Autodesk Inventor part; units mm, degrees
ref_plane "Startebene" through (0, 0, 0) normal (0, 0, 1) x (1, 0, 0)
ref_plane "Endebene" through (0, 0, 100) normal (0, 0, 1) x (1, 0, 0)
ref_plane "YZ Plane" through (0, 0, 0) normal (1, 0, 0) x (0, 1, 0)
ref_plane "Startebene" through (0, 0, 0) normal (0, 0, 1) x (1, 0, 0)
ref_plane "Endebene" through (0, 0, 100) normal (0, 0, 1) x (1, 0, 0)
sketch "Skizze" plane through (0, 0, 0) normal (0, 0, 1) x (1, 0, 0)
  arc A0 (-4.5287, -3.2559) -> (-3.65, -1.1346) centre (-6.65, -1.1346) ccw
  line L0 (-3.65, -1.1346) -> (-3.65, 1.1346)
  circle A1 centre (0, 0) radius 2.15
  line L1 (1.1346, -3.65) -> (-1.1346, -3.65)
  arc A2 (-1.1346, -3.65) -> (-3.2559, -4.5287) centre (-1.1346, -6.65) ccw
  line L2 (-6.779, -5.5062) -> (-4.5287, -3.2559)
  line L3 (-3.2559, -4.5287) -> (-5.5062, -6.779)
  arc A3 (-2.5, -8.5) -> (-2.8, -8.2) centre (-2.8, -8.5) ccw
  line L4 (-2.5, -8.5) -> (-2.5, -9.2)
  line L5 (-4.9176, -8.2) -> (-2.8, -8.2)
  arc A4 (-5.5062, -6.779) -> (-4.9176, -8.2) centre (-4.9176, -7.3676) ccw
  arc A5 (-3.3, -10) -> (-2.5, -9.2) centre (-3.3, -9.2) ccw
  line L6 (-3.3, -10) -> (-8, -10)
  line L7 (10, -3.3) -> (10, -8)
  line L8 (5.5062, -6.779) -> (3.2559, -4.5287)
  arc A6 (6.779, -5.5062) -> (8.2, -4.9176) centre (7.3676, -4.9176) ccw
  arc A7 (3.2559, -4.5287) -> (1.1346, -3.65) centre (1.1346, -6.65) ccw
  line L9 (4.5287, -3.2559) -> (6.779, -5.5062)
  arc A8 (3.65, -1.1346) -> (4.5287, -3.2559) centre (6.65, -1.1346) ccw
  arc A9 (8.5, -2.5) -> (8.2, -2.8) centre (8.5, -2.8) ccw
  line L10 (3.65, 1.1346) -> (3.65, -1.1346)
  line L11 (8.5, -2.5) -> (9.2, -2.5)
  arc A10 (10, -3.3) -> (9.2, -2.5) centre (9.2, -3.3) ccw
  line L12 (8.2, -4.9176) -> (8.2, -2.8)
  line L13 (2.5, 8.5) -> (2.5, 9.2)
  arc A11 (2.5, 8.5) -> (2.8, 8.2) centre (2.8, 8.5) ccw
  arc A12 (1.1346, 3.65) -> (3.2559, 4.5287) centre (1.1346, 6.65) ccw
  line L14 (-1.1346, 3.65) -> (1.1346, 3.65)
  arc A13 (3.3, 10) -> (2.5, 9.2) centre (3.3, 9.2) ccw
  line L15 (4.9176, 8.2) -> (2.8, 8.2)
  arc A14 (4.5287, 3.2559) -> (3.65, 1.1346) centre (6.65, 1.1346) ccw
  line L16 (3.2559, 4.5287) -> (5.5062, 6.779)
  arc A15 (5.5062, 6.779) -> (4.9176, 8.2) centre (4.9176, 7.3676) ccw
  line L17 (6.779, 5.5062) -> (4.5287, 3.2559)
  line L18 (3.3, 10) -> (8, 10)
  arc A16 (10, 8) -> (8, 10) centre (8, 8) ccw
  line L19 (8.2, 2.8) -> (8.2, 4.9176)
  line L20 (10, 8) -> (10, 3.3)
  arc A17 (8.2, 4.9176) -> (6.779, 5.5062) centre (7.3676, 4.9176) ccw
  line L21 (-2.8, 8.2) -> (-4.9176, 8.2)
  line L22 (-2.5, 9.2) -> (-2.5, 8.5)
  arc A18 (-2.5, 9.2) -> (-3.3, 10) centre (-3.3, 9.2) ccw
  arc A19 (-2.8, 8.2) -> (-2.5, 8.5) centre (-2.8, 8.5) ccw
  arc A20 (-3.65, 1.1346) -> (-4.5287, 3.2559) centre (-6.65, 1.1346) ccw
  arc A21 (-3.2559, 4.5287) -> (-1.1346, 3.65) centre (-1.1346, 6.65) ccw
  arc A22 (4.9176, -8.2) -> (5.5062, -6.779) centre (4.9176, -7.3676) ccw
  arc A23 (8, -10) -> (10, -8) centre (8, -8) ccw
  line L23 (2.8, -8.2) -> (4.9176, -8.2)
  line L24 (8, -10) -> (3.3, -10)
  arc A24 (2.8, -8.2) -> (2.5, -8.5) centre (2.8, -8.5) ccw
  arc A25 (2.5, -9.2) -> (3.3, -10) centre (3.3, -9.2) ccw
  line L25 (2.5, -9.2) -> (2.5, -8.5)
  arc A26 (8.2, 2.8) -> (8.5, 2.5) centre (8.5, 2.8) ccw
  line L26 (9.2, 2.5) -> (8.5, 2.5)
  arc A27 (9.2, 2.5) -> (10, 3.3) centre (9.2, 3.3) ccw
  arc A28 (-4.9176, 8.2) -> (-5.5062, 6.779) centre (-4.9176, 7.3676) ccw
  line L27 (-8, 10) -> (-3.3, 10)
  line L28 (-5.5062, 6.779) -> (-3.2559, 4.5287)
  arc A29 (-8, 10) -> (-10, 8) centre (-8, 8) ccw
  arc A30 (-6.779, 5.5062) -> (-8.2, 4.9176) centre (-7.3676, 4.9176) ccw
  line L29 (-10, 3.3) -> (-10, 8)
  line L30 (-8.2, 4.9176) -> (-8.2, 2.8)
  arc A31 (-8.5, 2.5) -> (-8.2, 2.8) centre (-8.5, 2.8) ccw
  line L31 (-8.5, 2.5) -> (-9.2, 2.5)
  arc A32 (-10, 3.3) -> (-9.2, 2.5) centre (-9.2, 3.3) ccw
  line L32 (-4.5287, 3.2559) -> (-6.779, 5.5062)
  line L33 (-10, -8) -> (-10, -3.3)
  arc A33 (-8.2, -4.9176) -> (-6.779, -5.5062) centre (-7.3676, -4.9176) ccw
  arc A34 (-10, -8) -> (-8, -10) centre (-8, -8) ccw
  line L34 (-10, -8) -> (-10, -3.3)
  arc A35 (-8.2, -2.8) -> (-8.5, -2.5) centre (-8.5, -2.8) ccw
  line L35 (-9.2, -2.5) -> (-8.5, -2.5)
  arc A36 (-9.2, -2.5) -> (-10, -3.3) centre (-9.2, -3.3) ccw
  line L36 (-8.2, -2.8) -> (-8.2, -4.9176)
  dimension "d4" = 4.3
  dimension "d5" = 6.35
  dimension "d6" = 10
  dimension "d7" = 2.5
  dimension "d8" = 5.8
  dimension "d9" = 10.5
  dimension "d10" = 3
  dimension "d11" = 7.5
  dimension "d12" = 12.5
  dimension "d13" = 13.65
  dimension "d14" = 5.7
  dimension "d15" = 10.7
  dimension "d16" = 1.15
  dimension "d17" = 6.15
  dimension "d18" = 1.8
  dimension "d19" = 0.8
  dimension "d20" = 0.3
  dimension "d21" = 2
  dimension "d22" = 0.8324
  dimension "d23" = 45
  dimension "d24" = 90
  dimension "d25" = 90
  dimension "d26" = 1.8
  dimension "d27" = 18.2
  dimension "d28" = 20
  dimension "d29" = 5
  dimension "d30" = 7.5
  dimension "d31" = 1.8
  dimension "d32" = 0.9
  dimension "d33" = 0.9
  dimension "d34" = 20
extrude "Körper" add sketch "Skizze" along normal up to surface (100 mm away) from surface at 0
sketch "Skizze6" plane through (0, 0, 0) normal (0, 0, 1) x (1, 0, 0)
  line L0 (0, 0) -> (10, 0)
ref_plane "Arbeitsebene4" through (0, 0, 0) normal (0, -1, 0) x (1, 0, 0)
sketch "Skizze7" plane through (0, 0, 0) normal (0, -1, 0) x (1, 0, 0)
  line L0 (-2, 0) -> (12, 0)
  line L1 (-2, 100) -> (12, 100)
  dimension "d43" = 100
equation "\"G_OFFSET_START\" = 0"
equation "\"G_OFFSET_END\" = 0"
equation "\"G_L\" = d43"
properties part number "BT001_trajan20_22"
For this review, take the finished solid that the model builds, in its own axes (mm). A direction names the side the tool comes from. Coordinates: 2 decimals unless noted, no trailing zeros. Order: outer loops, then holes, each group sorted by start corner. A loop starts at its lowest first (then second) coordinate and runs counter-clockwise, first axis right, second up. Notation, with made-up numbers: (10, -2) -> (27, -2) arc R23 cw to (27, 31) -> close; hole circle Ø11 at (-21.75, 7.25). An arc over 180 degrees is marked (long way). Answer as CSV lines item,"result".
Q1. For faces 4 (the face through (-10, 6, 49)), 5 (the face through (-3.65, 0, 49)), 6 (the face through (-0.1, 2.4, 0)), 7 (the face through (3.885, -2.298, 49.3)), 8 (the face through (3.65, 0, 49)), list the 3-axis set-ups (+Z, -Z, +X, -X, +Y, -Y) from which the entire face can be reached by the end or side of a thin tool; tool diameter is ignored.
Model answer:
face 4,"+Z, -Z, -X, +Y, -Y"
face 5,"+Z, -Z, -X"
face 6,"-Z, +X, -X, +Y, -Y"
face 7,"+Z, -Z"
face 8,"+Z, -Z, +X"
Q2. Wall thickness on line 1 along Y through (x, z) = (0, 71.5); line 2 along Y through (x, z) = (-7.25, 89.5); line 3 along Y through (x, z) = (-4.75, 50): over which ranges is each line inside the solid? List them lowest first. Write a range as [from, to].
Model answer:
line 1,"y = [-3.65, -2.15], [2.15, 3.65]"
line 2,"y = [-10, -5.74], [5.74, 10]"
line 3,"y = [-10, -8.2], [-6.02, -3.48], [3.48, 6.02], [8.2, 10]"
Q3. We need section A-A (y = 0). State the section outline as (x, z) points.
Model answer:
outline,"(-3.65, 0) -> (-2.15, 0) -> (-2.15, 100) -> (-3.65, 100) -> close; (2.15, 0) -> (3.65, 0) -> (3.65, 100) -> (2.15, 100) -> close"
Q4. Clearance check with flat-ended pins moving along their axes: pin 1 Ø0.8 at (x, z) = (8.5, 44) entering from +Y; pin 2 Ø0.6 at (x, z) = (-9, 48.5) entering from -Y; pin 3 Ø1 at (x, y) = (-5.5, -1.5) entering from -Z; pin 4 Ø0.6 at (y, z) = (9, 27.5) entering from -X. State where each tip first meets the part, or that it passes through.
Model answer:
pin 1,"stops at y = 10"
pin 2,"stops at y = -9.87"
pin 3,"passes through"
pin 4,"stops at x = -9.87"
Q5. Draft analysis for pull direction Y (two halves, no side actions). For faces 1 (the face through (-8.2, -4, 49)), 2 (the face through (10, -6, 49)), 3 (the face through (6, -10, 49)), state which applies: released by +Y, released by -Y, zero draft, split by the parting line, or undercut.
Model answer:
face 1,"undercut"
face 2,"zero draft"
face 3,"released by -Y"
